Can you work these out from the model? Positions are in its coordinate system, mm. A direction names the side the tool comes from. Give positions to 0.01 mm unless a question says otherwise; leave off trailing zeros. Write each loop counter-clockwise with the first axis right and the second up, starting at its lowest first coordinate (ties: lowest second). Pieces come first, ordered by that corner, then holes.
from build123d import *

# Parameters (mm, degrees)
SKETCH1_W           = 118.1
SKETCH1_H           = 128.6
BOSS_EXTRUDE2_DEPTH = 66.6
SKETCH5_R           = 2.4
CUT_EXTRUDE2_DEPTH  = 4
SKETCH4_W           = 6.3
SKETCH4_H           = 3.8
CUT_EXTRUDE3_DEPTH  = 4
SKETCH6_W           = 112.1
SKETCH6_H           = 122.6
CUT_EXTRUDE4_DEPTH  = 63.3
SKETCH9_W           = 125.5
SKETCH9_H           = 1.5
CUT_EXTRUDE7_DEPTH  = 115.5
SKETCH10_W          = 125.5
SKETCH10_H          = 1
CUT_EXTRUDE8_DEPTH  = 3.5


with BuildPart() as part:
    # Sketch1 → Boss-Extrude2 (new body)
    with BuildSketch(Plane(origin=(0, 0, 0), x_dir=(1, 0, 0), z_dir=(0, 1, 0))):
        Rectangle(SKETCH1_W, SKETCH1_H)
    extrude(amount=BOSS_EXTRUDE2_DEPTH)

    # Sketch5 → Cut-Extrude2 (cut)
    with BuildSketch(Plane(origin=(0, 0, -64.3), x_dir=(-1, 0, 0), z_dir=(0, 0, -1))):
        with Locations((43.05, 48.4)):
            Circle(SKETCH5_R)
        with Locations((4.65, 48.4)):
            Circle(SKETCH5_R)
        Polygon((9.65, 40), (38.05, 40), (38.05, 53.016960095), (32.8, 58.266960095), (14.4, 58.266960095), (9.65, 53.516960095), align=None)
    extrude(amount=-CUT_EXTRUDE2_DEPTH, mode=Mode.SUBTRACT)

    # Sketch4 → Cut-Extrude3 (cut)
    with BuildSketch(Plane.XY.offset(64.3)):
        with Locations((50.9, 5.9)):
            Rectangle(SKETCH4_W, SKETCH4_H)
        with Locations((40.9, 5.9)):
            Rectangle(SKETCH4_W, SKETCH4_H)
    extrude(amount=-CUT_EXTRUDE3_DEPTH, mode=Mode.SUBTRACT)

    # Sketch6 → Cut-Extrude4 (cut)
    with BuildSketch(Plane(origin=(0, 66.6, 0), x_dir=(1, 0, 0), z_dir=(0, 1, 0))):
        Rectangle(SKETCH6_W, SKETCH6_H)
    extrude(amount=-CUT_EXTRUDE4_DEPTH, mode=Mode.SUBTRACT)

    # Sketch9 → Cut-Extrude7 (cut)
    with BuildSketch(Plane(origin=(59.05, 0, 0), x_dir=(0, 0, -1), z_dir=(1, 0, 0))):
        with Locations((0.05, 65.35)):
            Rectangle(SKETCH9_W, SKETCH9_H)
    extrude(amount=-CUT_EXTRUDE7_DEPTH, mode=Mode.SUBTRACT)

    # Sketch10 → Cut-Extrude8 (cut)
    with BuildSketch(Plane(origin=(59.05, 0, 0), x_dir=(0, 0, -1), z_dir=(1, 0, 0))):
        with Locations((0.05, 66.1)):
            Rectangle(SKETCH10_W, SKETCH10_H)
    extrude(amount=-CUT_EXTRUDE8_DEPTH, mode=Mode.SUBTRACT)


solid = part.part
(1) Will this pin go through, and if not, where does the flat tip stop? P1, Ø5, axis at x = 26, z = 0.5, coming from the +Y side.
Returned:
P1: stops at y = 3.3
(2) Imagine slicing it at D-D, the plane z = 44. Write out the boundary of the cut face in (x, y), plus the area to 3 significant figures.
Returned:
outline: (-59.05, 0) - (59.05, 0) - (59.05, 64.6) - (56.05, 64.6) - (56.05, 3.3) - (-56.05, 3.3) - (-56.05, 64.6) - (-56.45, 64.6) - (-56.45, 66.1) - (-56.05, 66.1) - (-56.05, 66.6) - (-59.05, 66.6) - close
area: 763 mm2
(3) Imagine slicing it at B-B, the plane x = -43.05. Write out the boundary of the cut face in (y, z), plus the area to 3 significant figures.
Returned:
outline: (0, -64.3) - (46, -64.3) - (46, -61.3) - (3.3, -61.3) - (3.3, 61.3) - (64.6, 61.3) - (64.6, 62.7) - (66.1, 62.7) - (66.1, 61.3) - (66.6, 61.3) - (66.6, 64.3) - (0, 64.3) - close; (50.8, -64.3) - (66.6, -64.3) - (66.6, -61.3) - (66.1, -61.3) - (66.1, -62.8) - (64.6, -62.8) - (64.6, -61.3) - (50.8, -61.3) - close
area: 785 mm2
(4) If we mould it in two halves opening along X, with no side actions, what happens to faces 6 (the face through (-59.05, 33, 1)), 7 (the face through (-1, 33, 64.3)), 8 (the face through (54.05, 6, 63))? For each: +X half, -X half, draft (parallel to the pull), parting line (faces both ways), or undercut.
Returned:
face 6: -X half
face 7: draft
face 8: undercut
(5) For faces 1 (the face through (-1, 33, -64.3)), 2 (the face through (-1, 0, -1)), 3 (the face through (51, 7.8, 63)), 4 (the face through (-35.462, 55.605, -62.821)), 5 (the face through (-56.05, 34, 1)), which set-ups out of +Z, -Z, +X, -X, +Y, -Y let a thin tool reach every point of the face, with its end or its side?
Returned:
face 1: -Z, +X, -X, +Y, -Y
face 2: +Z, -Z, +X, -X, -Y
face 3: +Z
face 4: -Z
face 5: +Y
(6) Imagine slicing it at A-A, the plane y = 48.4. Write out the boundary of the cut face in (x, z), plus the area to 3 significant figures.
Returned:
outline: (-59.05, -64.3) - (-45.45, -64.3) - (-45.45, -61.3) - (-56.05, -61.3) - (-56.05, 61.3) - (56.05, 61.3) - (56.05, -61.3) - (-2.25, -61.3) - (-2.25, -64.3) - (59.05, -64.3) - (59.05, 64.3) - (-59.05, 64.3) - close; (-40.65, -64.3) - (-38.05, -64.3) - (-38.05, -61.3) - (-40.65, -61.3) - close; (-9.65, -64.3) - (-7.05, -64.3) - (-7.05, -61.3) - (-9.65, -61.3) - close
area: 1,330 mm2
(7) If I drill on L1, parallel to X at y = 48, z = -63; L2, parallel to Z at x = 42, y = 62; L3, parallel to X at y = 53, z = 8, over which ranges is the centre line in solid material (lowest first)?
Returned:
L1: x = -59.05 to -45.42, -40.68 to -38.05, -9.65 to -7.02, -2.28 to 59.05
L2: z = -64.3 to -61.3, 61.3 to 64.3
L3: x = -59.05 to -56.05, 56.05 to 59.05
(8) Imagine slicing it at C-C, the plane y = 10. Write out the boundary of the cut face in (x, z), plus the area to 3 significant figures.
Returned:
outline: (-59.05, -64.3) - (59.05, -64.3) - (59.05, 64.3) - (-59.05, 64.3) - close; hole (-56.05, -61.3) - (56.05, -61.3) - (56.05, 61.3) - (-56.05, 61.3) - close
area: 1,440 mm2
